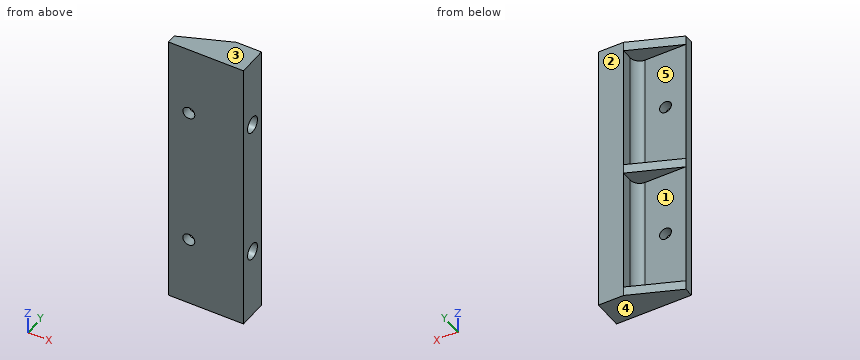
from build123d import *

# Parameters (mm, degrees)
BOSS_EXTRUDE1_DEPTH   = 90
RIB3_REACH            = 53.877
SKETCH4_WALL_W        = 123.024434014
SKETCH4_WALL_H        = 3
RIB4_START            = -3
RIB4_DEPTH            = 3
F_6_CLEARANCE_HOLE1_D = 3.7973
SKETCH6_R             = 2.3495
CUT_EXTRUDE1_DEPTH    = 7
SKETCH12_R            = 2.6162
CUT_EXTRUDE2_DEPTH    = 6.35


# Read off the part's stored shape, not the designer's step: Rib4
with BuildPart() as part:
    # Sketch1 → Boss-Extrude1 (new body)
    with BuildSketch(Plane.XY):
        with BuildLine():
            Line((0, 0), (0, 9.5))
            Line((0, 9.5), (-8, 9.5))
            Line((-8, 9.5), (-8, 6))
            ThreePointArc((-8, 6), (-8.878679656, 3.878679656), (-11, 3))
            Line((-11, 3), (-24, 3))
            Line((-24, 3), (-24, 0))
            Line((-24, 0), (0, 0))
        make_face()
    extrude(amount=BOSS_EXTRUDE1_DEPTH)

    # Sketch4 wall → Rib3 (add, up to next)
    with BuildSketch(Plane(origin=(-16, 6.25, 45), x_dir=(-0.926466577122, -0.376377046956, 0), z_dir=(-0.376377046956, 0.926466577122, 0)), mode=Mode.PRIVATE) as rib3_sk1:
        Rectangle(SKETCH4_WALL_W, SKETCH4_WALL_H)
    rib3_tool1 = extrude(rib3_sk1.sketch, amount=-RIB3_REACH, mode=Mode.PRIVATE) - part.part
    add(rib3_tool1.solids().sort_by_distance((-16, 6.25, 45))[0])

    # Rib4 outline → Rib4 (add)
    with BuildSketch(Plane(origin=(0, 0, 0), x_dir=(-1, 0, 0), z_dir=(0, 0, -1)).offset(RIB4_START)):
        with BuildLine():
            Line((24, 3), (8, 9.5))
            Line((8, 9.5), (8, 6))
            ThreePointArc((8, 6), (8.878679656, 3.878679656), (11, 3))
            Line((11, 3), (24, 3))
        make_face()
    rib4 = extrude(amount=RIB4_DEPTH)

    # Mirror1: Rib4 across plane
    add(rib4.mirror(Plane(origin=(0, 0, 45), x_dir=(1, 0, 0), z_dir=(0, 0, -1))))

    # #6 Clearance Hole1 (through all)
    with Locations(Plane(origin=(0, 0, 0), x_dir=(-1, 0, 0), z_dir=(0, -1, 0))):
        with Locations((17.5, -22.5), (17.5, -67.5)):
            Hole(F_6_CLEARANCE_HOLE1_D / 2)

    # Sketch6 → Cut-Extrude1 (cut)
    with BuildSketch(Plane(origin=(0, 0, 0), x_dir=(0, 0, -1), z_dir=(1, 0, 0))):
        with Locations((-67.5, 4.75)):
            Circle(SKETCH6_R)
        with Locations((-22.5, 4.75)):
            Circle(SKETCH6_R)
    extrude(amount=-CUT_EXTRUDE1_DEPTH, mode=Mode.SUBTRACT)

    # Sketch12 → Cut-Extrude2 (cut)
    with BuildSketch(Plane(origin=(0, 0, 0), x_dir=(0, 0, -1), z_dir=(1, 0, 0))):
        with Locations((-67.5, 4.75)):
            Circle(SKETCH12_R)
        with Locations((-22.5, 4.75)):
            Circle(SKETCH12_R)
    extrude(amount=-CUT_EXTRUDE2_DEPTH, mode=Mode.SUBTRACT)


solid = part.part
The model under review builds one solid part; all positions refer to its coordinate system, in mm. Face numbers are marked on the shaded views. A direction names the side the tool comes from. Coordinates: 2 decimals unless noted, no trailing zeros. Loops run counter-clockwise (first coordinate to the right, second up) from the corner with the lowest first, then second, coordinate; pieces in that order, holes last.
(1) Draft analysis for pull direction Z (two halves, no side actions). For the marked faces 1, 2 and 3, state which applies: +Z half, -Z half, draft (parallel to the pull), parting line (faces both ways), or undercut.
Determined:
face 1: undercut
face 2: draft
face 3: +Z half
(2) Insertion check: P1, Ø4, axis at y = 4.75, z = 67.5, coming from the +X side; P2, Ø4, axis at y = 7, z = 15.5, coming from the -X side; P3, Ø4, axis at x = -16, z = 66.5, coming from the +Y side. Each pin has a flat end and moves straight along its axis. Give the tip position at first contact, or say it passes through.
Determined:
P1: stops at x = -7
P2: stops at x = -8.17
P3: stops at y = 3
(3) Wall thickness on L1, parallel to X at y = 1.9, z = 22.5; L2, parallel to Z at x = -12.25, y = 5.25; L3, parallel to Y at x = -4.25, z = 22.5: over which ranges is each line inside the solid? List them lowest first.
Determined:
L1: x = -24 to -19.4, -15.6 to 0
L2: z = 0 to 3, 43.5 to 46.5, 87 to 90
L3: y = 0 to 2.13, 7.37 to 9.5
(4) Consider section C-C, the plane x = -17.5. Give the boundary of the cut face in (y, z).
Determined:
outline: (0, 0) - (5.64, 0) - (5.64, 3) - (3, 3) - (3, 20.6) - (0, 20.6) - close; (0, 24.4) - (3, 24.4) - (3, 43.5) - (5.64, 43.5) - (5.64, 46.5) - (3, 46.5) - (3, 65.6) - (0, 65.6) - close; (0, 69.4) - (3, 69.4) - (3, 87) - (5.64, 87) - (5.64, 90) - (0, 90) - close
(5) Consider section D-D, the plane y = 4.75. Give the boundary of the cut face in (x, z), plus the area to 3 significant figures.
Determined:
outline: (-19.69, 0) - (0, 0) - (0, 19.88) - (-6.35, 19.88) - (-6.35, 20.15) - (-7, 20.15) - (-7, 24.85) - (-6.35, 24.85) - (-6.35, 25.12) - (0, 25.12) - (0, 64.88) - (-6.35, 64.88) - (-6.35, 65.15) - (-7, 65.15) - (-7, 69.85) - (-6.35, 69.85) - (-6.35, 70.12) - (0, 70.12) - (0, 90) - (-19.69, 90) - (-19.69, 87) - (-8.27, 87) - (-8.27, 46.5) - (-19.69, 46.5) - (-19.69, 43.5) - (-8.27, 43.5) - (-8.27, 3) - (-19.69, 3) - close
area: 775 mm2
(6) Consider section A-A, the plane z = 22.5. Give the boundary of the cut face in (x, y).
Determined:
outline: (-24, 0) - (-19.4, 0) - (-19.4, 3) - (-24, 3) - close; (-15.6, 0) - (0, 0) - (0, 2.13) - (-6.35, 2.13) - (-6.35, 2.4) - (-7, 2.4) - (-7, 7.1) - (-6.35, 7.1) - (-6.35, 7.37) - (0, 7.37) - (0, 9.5) - (-8, 9.5) - (-8, 6) arc R3 cw to (-11, 3) - (-15.6, 3) - close
(7) Consider section B-B, the plane x = -1.5. Give the boundary of the cut face in (y, z).
Determined:
outline: (0, 0) - (9.5, 0) - (9.5, 90) - (0, 90) - close; hole circle Ø5.23 at (4.75, 22.5); hole circle Ø5.23 at (4.75, 67.5)
(8) Tool access review of the marked faces 4 and 5: name each direction out of +Z, -Z, +X, -X, +Y, -Y from which nothing blocks a thin tool from reaching the whole face with its end or side.
Determined:
face 4: -Z, +X, -X, +Y, -Y
face 5: -X, +Y
